from build123d import *

# Parameters (mm, degrees)
SKETCH2_R               = 10
BOSS_EXTRUDE1_DEPTH     = 18
SKETCH5_R               = 4
CUT_EXTRUDE1_DEPTH      = 18
CUT_EXTRUDE1_DEPTH_BACK = 21
SKETCH6_OUTSIDE_W       = 28.706
SKETCH6_OUTSIDE_H       = 28.706
SKETCH6_OUTSIDE_R       = 8.042126696
CUT_EXTRUDE2_DEPTH      = 24
SKETCH8_R               = 6.210271538
CUT_EXTRUDE4_DEPTH      = 15
FILLET1_R               = 1


with BuildPart() as part:
    # Sketch2 → Boss-Extrude1 (new body)
    with BuildSketch(Plane.XY):
        Circle(SKETCH2_R)
    extrude(amount=BOSS_EXTRUDE1_DEPTH)

    # Sketch5 → Cut-Extrude1 (cut, two sides)
    with BuildSketch(Plane(origin=(0, 0, 0), x_dir=(0, 0, -1), z_dir=(1, 0, 0))) as cut_extrude1_sk:
        with Locations((-9.266027008, 0)):
            Circle(SKETCH5_R)
    extrude(amount=CUT_EXTRUDE1_DEPTH, mode=Mode.SUBTRACT)
    extrude(cut_extrude1_sk.sketch, amount=-CUT_EXTRUDE1_DEPTH_BACK, mode=Mode.SUBTRACT)

    # Sketch6 outside → Cut-Extrude2 (cut)
    with BuildSketch(Plane(origin=(0, 0, 0), x_dir=(-1, 0, 0), z_dir=(0, 0, -1))):
        Rectangle(SKETCH6_OUTSIDE_W, SKETCH6_OUTSIDE_H)
        Circle(SKETCH6_OUTSIDE_R, mode=Mode.SUBTRACT)
    extrude(amount=-CUT_EXTRUDE2_DEPTH, mode=Mode.SUBTRACT)

    # Sketch8 → Cut-Extrude4 (cut)
    with BuildSketch(Plane.XY.offset(18)):
        Circle(SKETCH8_R)
    extrude(amount=-CUT_EXTRUDE4_DEPTH, mode=Mode.SUBTRACT)

    # Fillet1
    fillet1_edges = [part.edges().sort_by_distance(p)[0] for p in [
        (-6.210271538, 0, 3),
    ]]
    fillet(fillet1_edges, radius=FILLET1_R)


solid = part.part
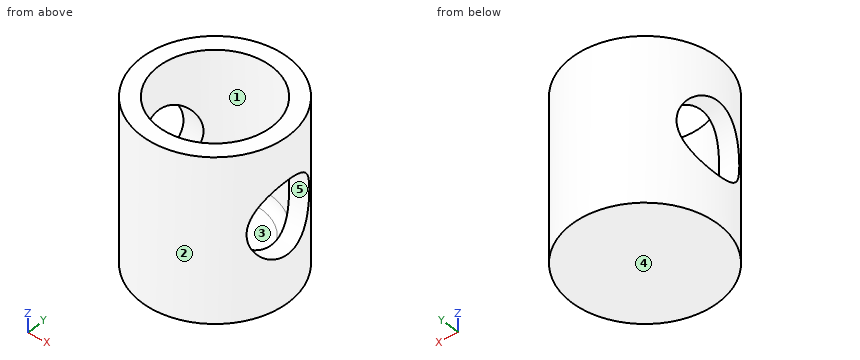
Model file for the job. Use its own axes, mm. Face numbers are marked on the shaded views. A direction names the side the tool comes from. Give positions to 0.01 mm unless a question says otherwise; leave off trailing zeros. Loops run counter-clockwise (first coordinate to the right, second up) from the corner with the lowest first, then second, coordinate; pieces in that order, holes last. Notation, with made-up numbers: (-12, -1.75) -> (30, -1.75) arc R21 ccw to (30, 36.25) -> close; hole circle Ø8 at (48.5, 65). An arc over 180 degrees is marked (long way). Use a Markdown table: item, result. Add a question column.
(1) Slice it at D-D on x = 0. List the corners of the cut face in (y, z).
(2) Wall check: line 1 along Z through (x, y) = (-6.8, 0); line 2 along X through (y, z) = (-0.25, 13.5); line 3 along Y through (x, z) = (0.75, 8). Give the ranges that are in metal, low to high.
(3) Tool access for the marked faces 1 and 2: list every direction of +Z, -Z, +X, -X, +Y, -Y with a clear straight run to the whole face (end or side of a thin tool).
(4) Drop flat-ended pins along their axis: pin 1 Ø1 at (x, y) = (-2, 3.5) entering from +Z; pin 2 Ø6.5 at (y, z) = (0, 9.27) entering from -X; pin 3 Ø8 at (y, z) = (-0.5, 8) entering from +X; pin 4 Ø6 at (y, z) = (1, 8.5) entering from -X. Give the stop position or say it passes through.
(5) Slice it at A-A on y = 0. List the corners of the cut face in (x, z).
(6) Slice it at C-C on z = 11.25. List the corners of the cut face in (x, y), and give its area (3 significant figures).
(7) Slice it at B-B on x = 7. List the corners of the cut face in (y, z).
(8) Mould opens along Z. For the marked faces 3, 4 and 5 say: +Z half, -Z half, draft (parallel to the pull), parting line (faces both ways), or undercut.
Filled sheet:
| question | item | result |
|---|---|---|
| 1 | outline | (-8.04, 0) -> (8.04, 0) -> (8.04, 18) -> (6.21, 18) -> (6.21, 4) arc R1 cw to (5.21, 3) -> (-5.21, 3) arc R1 cw to (-6.21, 4) -> (-6.21, 18) -> (-8.04, 18) -> close |
| 2 | line 1 | 0 to 5.27, 13.27 to 18 |
| 2 | line 2 | -8.04 to -6.21, 6.21 to 8.04 |
| 2 | line 3 | -8.01 to -6.16, 6.16 to 8.01 |
| 3 | face 1 | +Z |
| 3 | face 2 | +Z, -Z |
| 4 | pin 1 | z = 3 |
| 4 | pin 2 | through |
| 4 | pin 3 | x = 8.04 |
| 4 | pin 4 | x = -7.91 |
| 5 | outline | (-8.04, 0) -> (8.04, 0) -> (8.04, 5.27) -> (6.21, 5.27) -> (6.21, 4) arc R1 cw to (5.21, 3) -> (-5.21, 3) arc R1 cw to (-6.21, 4) -> (-6.21, 5.27) -> (-8.04, 5.27) -> close; (-8.04, 13.27) -> (-6.21, 13.27) -> (-6.21, 18) -> (-8.04, 18) -> close; (6.21, 13.27) -> (8.04, 13.27) -> (8.04, 18) -> (6.21, 18) -> close |
| 6 | outline | (-7.25, -3.47) arc R8.04 ccw to (7.25, -3.47) -> (5.15, -3.47) arc R6.21 cw to (-5.15, -3.47) -> close; (-7.25, 3.47) -> (-5.15, 3.47) arc R6.21 cw to (5.15, 3.47) -> (7.25, 3.47) arc R8.04 ccw to start |
| 6 | area | 55.4 mm2 |
| 7 | outline | (-3.96, 0) -> (3.96, 0) -> (3.96, 8.7) arc R4 cw to (-3.96, 8.7) -> close; (-3.96, 9.84) arc R4 cw to (3.96, 9.84) -> (3.96, 18) -> (-3.96, 18) -> close |
| 8 | face 3 | +Z half |
| 8 | face 4 | -Z half |
| 8 | face 5 | undercut |
